Could you check a few things on this model? Use its own coordinates, in mm. A direction names the side the tool comes from. Give positions to 0.01 mm unless a question says otherwise; leave off trailing zeros. Answer as CSV lines item,"result". Start each with the question number.
(1) I need wall thicknesses on L1, parallel to X at y = 55, z = 7; L2, parallel to Y at x = 58, z = 9.5; L3, parallel to X at y = 52, z = 10.5. Which ranges of each line are inside material? Lowest first, please.
(2) We'd pull the mould along X, two halves only. Please class faces 4 (the face through (17.509, 35.854, 14.617)), 5 (the face through (-50.52, 57.46, 13.06)), 6 (the face through (19.77, 25.11, 8.15)): released by +X, released by -X, zero draft, split by the parting line, or undercut.
(3) Will these pins go through, and if not, where does the flat tip stop? pin 1 Ø6 at (y, z) = (48.5, 11.5) entering from -X; pin 2 Ø1.5 at (x, z) = (31, 4) entering from +Y; pin 3 Ø3 at (x, y) = (-39.5, 36) entering from +Z (3 decimals).
(4) On a 3-axis mill with a long thin cutter (end or side, diameter ignored), from which of +Z, -Z, +X, -X, +Y, -Y can I reach the whole of each face in a straight line? I mean faces 1 (the face through (39, 58, 9)), 2 (the face through (51.06, 71.28, 13.06)), 3 (the face through (-18.183, 36.42, 14.617)). Say none if no direction works.
```python
from build123d import *

# Parameters (mm, degrees)
CHAMFER_1_SIZE      = 10
CHAMFER_1_SIZE_2    = 22.360679775
FILLET_3_R          = 5
CUT_EXTRUDE_START   = 5
CUT_EXTRUDE_2_DEPTH = 108.268120159
CUT_EXTRUDE_3_DEPTH = 108.268120141


with BuildPart() as part:
    # 草图1 → 放样1 section 0
    with BuildSketch(Plane.XY):
        with BuildLine():
            Line((0, 74), (70, 86.34288865))
            Line((70, 86.34288865), (70, 58.736974182))
            Line((70, 58.736974182), (0, 0))
            Line((0, 0), (-70, 58.736974182))
            Line((-70, 58.736974182), (-70, 86.34288865))
            Line((-70, 86.34288865), (0, 74))
        make_face()
    # 草图2 → 放样1 section 1
    with BuildSketch(Plane.XY.offset(20)):
        with BuildLine():
            Line((60, 74.425352724), (0, 63.845733881))
            Line((0, 63.845733881), (-60, 74.425352724))
            Line((-60, 74.425352724), (-60, 63.400050764))
            Line((-60, 63.400050764), (0, 13.054072893))
            Line((0, 13.054072893), (60, 63.400050764))
            Line((60, 63.400050764), (60, 74.425352724))
        make_face()
    loft()

    # 倒角1
    # the kernel refuses this chamfer: 22.360679775, 10 mm, written as the material it takes off along each edge
    with BuildSketch(Plane(origin=(57.145762753, 53.769394075, 20), x_dir=(0.07765782588644504, 0.44041941610082364, -0.8944271909999159), z_dir=(-0.9848077530122075, 0.17364817766693405, 0))) as chamfer_1_piece_1_section:
        Polygon((CHAMFER_1_SIZE, 0), (-CHAMFER_1_SIZE_2 * 0.4472135955, CHAMFER_1_SIZE_2 * 0.894427191), (0, 0), align=None)
    chamfer_1_piece_1 = extrude(amount=176.980253225, mode=Mode.PRIVATE)
    chamfer_1_piece_1 = split(chamfer_1_piece_1, bisect_by=Plane(origin=(57.189420764, 53.521797191, 19.245750606), z_dir=(-0.05491237529650921, 0.3114235556911101, 0.9486832980505147)), keep=Keep.TOP, mode=Mode.PRIVATE)
    add(chamfer_1_piece_1, mode=Mode.SUBTRACT)
    with BuildSketch(Plane(origin=(117.145762753, 84.50169253, 20), x_dir=(-0.0776578258864451, 0.4404194161008233, -0.8944271909999161), z_dir=(-0.9848077530122074, -0.1736481776669343, 0))) as chamfer_1_piece_2_section:
        Polygon((CHAMFER_1_SIZE, 0), (-CHAMFER_1_SIZE_2 * 0.4472135955, CHAMFER_1_SIZE_2 * 0.894427191), (0, 0), align=None)
    chamfer_1_piece_2 = extrude(amount=176.980253225, mode=Mode.PRIVATE)
    chamfer_1_piece_2 = split(chamfer_1_piece_2, bisect_by=Plane(origin=(116.05099823, 78.292974393, 1.086507133), z_dir=(0.054912375296509185, 0.31142355569111035, 0.9486832980505147)), keep=Keep.TOP, mode=Mode.PRIVATE)
    add(chamfer_1_piece_2, mode=Mode.SUBTRACT)
    with BuildSketch(Plane(origin=(-44.451512359, -24.245174733, 20), x_dir=(0.28746335807073986, -0.34258548972000163, -0.894427190999916), z_dir=(0.7660444431189795, 0.6427876096865376, 0)), Plane(origin=(-104.451512359, 100.69929839, 20), x_dir=(-0.28746335807074064, -0.3425854897200026, -0.8944271909999154), z_dir=(0.7660444431189795, -0.6427876096865376, 0))) as chamfer_1_piece_3:
        Polygon((CHAMFER_1_SIZE, 0), (-CHAMFER_1_SIZE_2 * 0.4472135955, CHAMFER_1_SIZE_2 * 0.894427191), (0, 0), align=None)
    extrude(amount=194.379093872, mode=Mode.SUBTRACT)

    # 圆角3
    fillet_3_edges = [part.edges().sort_by_distance(p)[0] for p in [
        (-67.236067978, 60.025816851, 5.527864045),
        (-67.236067978, 83.048962732, 5.527864045),
        (67.236067977, 60.025816851, 5.527864045),
        (67.236067977, 83.048962732, 5.527864045),
    ]]
    fillet(fillet_3_edges, radius=FILLET_3_R)

    # 草图7 → 切除-拉伸2 (cut, through all)
    with BuildSketch(Plane.XY.offset(CUT_EXTRUDE_START)):
        Polygon((-40, 75.43993897), (-40, 40.780099266), (0, 7.216114019), (40, 40.780099266), (40, 75.43993897), (0, 68.386859742), align=None)
        Polygon((-39, 74.248185378), (0, 67.37143313), (39, 74.248185378), (39, 41.246406924), (0, 8.521521308), (-39, 41.246406924), align=None, mode=Mode.SUBTRACT)
    extrude(amount=CUT_EXTRUDE_2_DEPTH, mode=Mode.SUBTRACT)

    # 草图9 → 切除-拉伸3 (cut, through all)
    with BuildSketch(Plane.XY.offset(CUT_EXTRUDE_START)):
        with BuildLine():
            Line((-40, 75.43993897), (0, 68.386859742))
            Line((0, 68.386859742), (40, 75.43993897))
            Line((40, 75.43993897), (59.223421741, 78.829546885))
            add(Edge.make_bspline(
                [(63.422393112, 73.174317919), (64.472135955, 79.755036815), (59.223421741, 78.829546885)],
                knots=[2.124820971, 2.124820971, 2.124820971, 3.634497794, 3.634497794, 3.634497794], degree=2, weights=[1, 0.728382268, 1]))
            Line((63.422393112, 73.174317919), (63.081692851, 71.038506602))
            Line((63.081692851, 71.038506602), (64.15263548, 63.549036282))
            add(Edge.make_bspline(
                [(62.874633581, 59.974195867), (64.472135955, 61.31465952), (64.15263548, 63.549036282)],
                knots=[2.89691376, 2.89691376, 2.89691376, 3.672186613, 3.672186613, 3.672186613], degree=2, weights=[1, 0.925805079, 1]))
            Line((62.874633581, 59.974195867), (40, 40.780099266))
            Line((40, 40.780099266), (0, 7.216114019))
            Line((0, 7.216114019), (-40, 40.780099266))
            Line((-40, 40.780099266), (-62.874633581, 59.974195867))
            add(Edge.make_bspline(
                [(-64.15263548, 63.549036282), (-64.472135955, 61.31465952), (-62.874633581, 59.974195867)],
                knots=[2.610998694, 2.610998694, 2.610998694, 3.386271547, 3.386271547, 3.386271547], degree=2, weights=[1, 0.925805079, 1]))
            Line((-64.15263548, 63.549036282), (-63.081692851, 71.038506602))
            Line((-63.081692851, 71.038506602), (-63.422393112, 73.174317919))
            add(Edge.make_bspline(
                [(-59.223421741, 78.829546885), (-64.472135955, 79.755036815), (-63.422393112, 73.174317919)],
                knots=[2.648687513, 2.648687513, 2.648687513, 4.158364336, 4.158364336, 4.158364336], degree=2, weights=[1, 0.728382268, 1]))
            Line((-59.223421741, 78.829546885), (-40, 75.43993897))
        make_face()
        with BuildLine():
            Line((-59.31024583, 78.337143008), (-40.086824089, 74.947535094))
            Line((-40.086824089, 74.947535094), (0, 67.879146436))
            Line((0, 67.879146436), (40.086824089, 74.947535094))
            Line((40.086824089, 74.947535094), (59.31024583, 78.337143008))
            add(Edge.make_bspline(
                [(59.31024583, 78.337143008), (59.606035397, 78.389298689), (60.236089665, 78.427658938), (61.023214098, 78.258065344), (61.707637648, 77.888235871), (62.45863279, 77.130661919), (62.942544445, 75.958588793), (63.064569227, 74.489707699), (62.992457265, 73.653171126), (62.92863572, 73.253081091)],
                knots=[2.124820971, 2.124820971, 2.124820971, 2.124820971, 2.313530574, 2.502240177, 2.69094978, 2.879659382, 3.257078588, 3.445788191, 3.634497794, 3.634497794, 3.634497794, 3.634497794], degree=3))
            Line((62.92863572, 73.253081091), (62.576022888, 71.04259122))
            Line((62.576022888, 71.04259122), (63.657670159, 63.478259653))
            add(Edge.make_bspline(
                [(63.657670159, 63.478259653), (63.701203567, 63.173815556), (63.721909403, 62.536225056), (63.535721886, 61.698867433), (63.156823887, 60.958692701), (62.768132959, 60.537534879), (62.553239776, 60.357218088)],
                knots=[2.89691376, 2.89691376, 2.89691376, 2.89691376, 3.090731973, 3.284550187, 3.4783684, 3.672186613, 3.672186613, 3.672186613, 3.672186613], degree=3))
            Line((62.553239776, 60.357218088), (39.678606195, 41.163121487))
            Line((39.678606195, 41.163121487), (0, 7.868817663))
            Line((0, 7.868817663), (-39.678606195, 41.163121487))
            Line((-39.678606195, 41.163121487), (-62.553239776, 60.357218088))
            add(Edge.make_bspline(
                [(-62.553239776, 60.357218088), (-62.768132959, 60.537534879), (-63.156823887, 60.958692701), (-63.535721886, 61.698867433), (-63.721909403, 62.536225056), (-63.701203567, 63.173815556), (-63.657670159, 63.478259653)],
                knots=[2.610998694, 2.610998694, 2.610998694, 2.610998694, 2.804816907, 2.998635121, 3.192453334, 3.386271547, 3.386271547, 3.386271547, 3.386271547], degree=3))
            Line((-63.657670159, 63.478259653), (-62.576022888, 71.04259122))
            Line((-62.576022888, 71.04259122), (-62.92863572, 73.253081091))
            add(Edge.make_bspline(
                [(-62.92863572, 73.253081091), (-62.992457265, 73.653171126), (-63.064569227, 74.489707699), (-62.942544445, 75.958588793), (-62.45863279, 77.130661919), (-61.707637648, 77.888235871), (-61.023214098, 78.258065344), (-60.236089665, 78.427658938), (-59.606035397, 78.389298689), (-59.31024583, 78.337143008)],
                knots=[2.648687513, 2.648687513, 2.648687513, 2.648687513, 2.837397116, 3.026106719, 3.403525925, 3.592235528, 3.78094513, 3.969654733, 4.158364336, 4.158364336, 4.158364336, 4.158364336], degree=3))
        make_face(mode=Mode.SUBTRACT)
    extrude(amount=CUT_EXTRUDE_3_DEPTH, mode=Mode.SUBTRACT)


solid = part.part
```
Final values:
1,L1,"-60.1 to -56.95, -56.17 to -40, -39 to 39, 40 to 56.17, 56.95 to 60.1"
1,L2,"54.87 to 55.88, 56.54 to 78.11, 78.61 to 79.4"
1,L3,"-53.8 to -53.37, -52.59 to -40, -39 to 39, 40 to 52.59, 53.37 to 53.8"
2,face 4,"released by +X"
2,face 5,"released by -X"
2,face 6,"undercut"
3,pin 1,"x = -53.12"
3,pin 2,"y = 77.84"
3,pin 3,"z = 7.375"
4,face 1,"+Z"
4,face 2,"+Z, +Y"
4,face 3,"+Z, -X, -Y"
